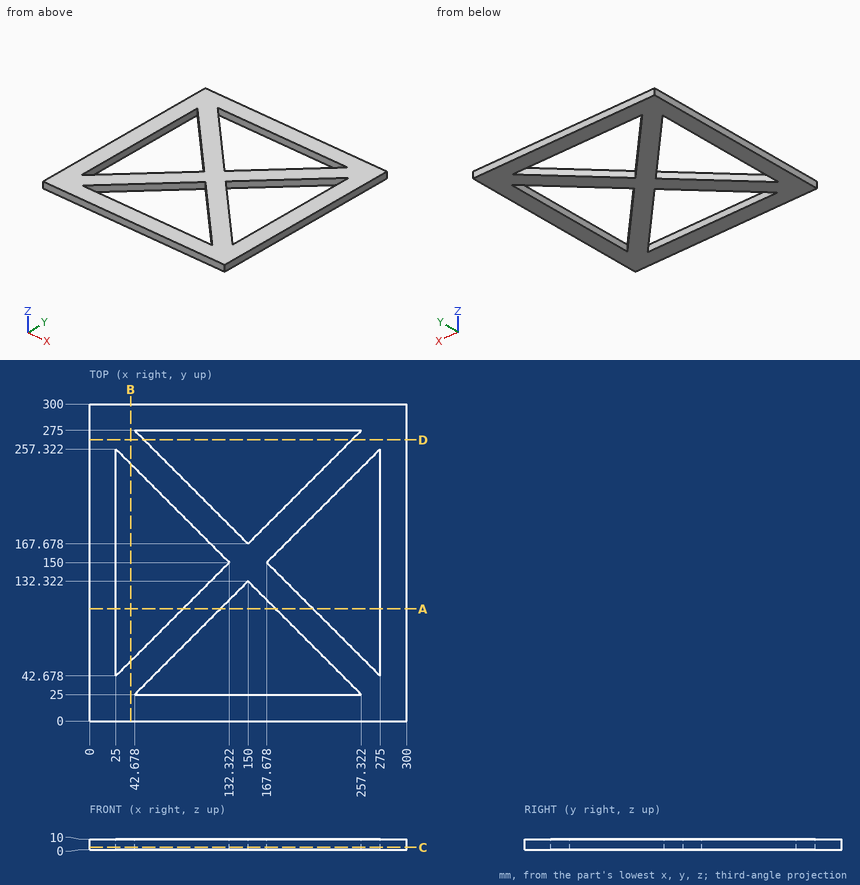
Input: dimensioned drawing with shaded views. Units: mm. Origin: part minimum x, y, z. Coordinates: 2 decimals unless noted, no trailing zeros. Loops run counter-clockwise (first coordinate to the right, second up) from the corner with the lowest first, then second, coordinate; pieces in that order, holes last.
Q1. Line query: line 1 along X through (y, z) = (231.5, 3.25); line 2 along X through (y, z) = (52, 6); line 3 along Y through (x, z) = (134, 7). Output: solid intervals per line, ascending.
Results are:
line 1: x = 0 to 25, 50.82 to 86.18, 213.82 to 249.18, 275 to 300
line 2: x = 0 to 25, 34.32 to 69.68, 230.32 to 265.68, 275 to 300
line 3: y = 0 to 25, 116.32 to 183.68, 275 to 300
Q2. Section B-B, the plane x = 39. Return the cut outline in (y, z).
Results are:
outline: (0, 0) - (56.68, 0) - (56.68, 10) - (0, 10) - close; (243.32, 0) - (300, 0) - (300, 10) - (243.32, 10) - close
Q3. Contact query for a flat-ended pin moving along its axis: pin 1 (6 mm diameter, centred on y = 195.5, z = 3.5, fed in from -X). Output: stop coordinate, or through.
Results are:
pin 1: stops at x = 0
Q4. Section D-D, the plane y = 266. Return the cut outline in (x, z), and give its area (3 significant figures).
Results are:
outline: (0, 0) - (51.68, 0) - (51.68, 10) - (0, 10) - close; (248.32, 0) - (300, 0) - (300, 10) - (248.32, 10) - close
area: 1,030 mm2
Q5. Section A-A, the plane y = 106. Return the cut outline in (x, z), and give its area (3 significant figures).
Results are:
outline: (0, 0) - (25, 0) - (25, 10) - (0, 10) - close; (88.32, 0) - (123.68, 0) - (123.68, 10) - (88.32, 10) - close; (176.32, 0) - (211.68, 0) - (211.68, 10) - (176.32, 10) - close; (275, 0) - (300, 0) - (300, 10) - (275, 10) - close
area: 1,210 mm2
Q6. Section C-C, the plane z = 2. Return the cut outline in (x, y).
Results are:
outline: (0, 0) - (300, 0) - (300, 300) - (0, 300) - close; hole (25, 42.68) - (132.32, 150) - (25, 257.32) - close; hole (42.68, 25) - (257.32, 25) - (150, 132.32) - close; hole (42.68, 275) - (150, 167.68) - (257.32, 275) - close; hole (167.68, 150) - (275, 42.68) - (275, 257.32) - close
